Design review of the part built by this model. Coordinates are the model's own, in mm. A direction names the side the tool comes from. Coordinates: 2 decimals unless noted, no trailing zeros. Order: outer loops, then holes, each group sorted by start corner. A loop starts at its lowest first (then second) coordinate and runs counter-clockwise, first axis right, second up. Notation, with made-up numbers: (-38.5, 46.25) - (4.5, 46.25) arc R21 cw to (4.5, 76.25) - close; hole circle Ø6 at (55.5, -20.5). An arc over 180 degrees is marked (long way). Write each question's results on one line, items separated by ' | '. Start each with the question number.
Autodesk Inventor part; units mm, degrees
ref_plane "Work Plane1" through (0, 0, 5) normal (0, 0, 1) x (1, 0, 0)
ref_plane "YZ Plane" through (0, 0, 0) normal (1, 0, 0) x (0, 1, 0)
ref_plane "XZ Plane" through (0, 0, 0) normal (0, 1, 0) x (-1, 0, 0)
sketch "Sketch1" plane through (0, 0, 0) normal (0, 0, 1) x (1, 0, 0)
  line L0 (-5.8474, 0) -> (5.8474, 0) construction
  line L1 (2.5, 18.75) -> (7.5, 18.75)
  line L2 (7.5, 18.75) -> (7.5, 37.5)
  line L3 (7.5, 37.5) -> (-7.5, 37.5)
  line L4 (-7.5, 37.5) -> (-7.5, 18.75)
  line L5 (-7.5, 18.75) -> (2.5, 18.75)
  circle A0 centre (3.75, 33.75) radius 1.6
  circle A1 centre (-3.75, 33.75) radius 1.6
  line L6 (2.5, -18.75) -> (7.5, -18.75)
  line L7 (7.5, -18.75) -> (7.5, -37.5)
  line L8 (7.5, -37.5) -> (-7.5, -37.5)
  line L9 (-7.5, -37.5) -> (-7.5, -18.75)
  line L10 (-7.5, -18.75) -> (2.5, -18.75)
  circle A2 centre (3.75, -33.75) radius 1.6
  circle A3 centre (-3.75, -33.75) radius 1.6
  line L11 (7.5, 28.125) -> (27.5, 8.125)
  line L12 (7.5, 28.125) -> (35.7843, 28.125) construction
  line L13 (2.5, 18.75) -> (12.5, 8.75)
  line L14 (12.5, 8.75) -> (12.5, 0)
  line L15 (27.5, 8.125) -> (27.5, 0)
  line L16 (7.5, -28.125) -> (27.5, -8.125)
  line L17 (2.5, -18.75) -> (12.5, -8.75)
  line L18 (12.5, -8.75) -> (12.5, 0)
  line L19 (27.5, -8.125) -> (27.5, 0)
  point P0 (0, 0)
  point P1 (0, 0)
  point P2 (2.5, -18.75)
  point P3 (2.5, -18.75)
  point P4 (2.5, 18.75)
  dimension "d2" = 15
  dimension "d3" = 18.75
  dimension "d4" = 7.5
  dimension "d5" = 3.2
  dimension "d6" = 3.2
  dimension "d7" = 3.75
  dimension "d8" = 3.75
  dimension "d9" = 7.5
  dimension "d10" = 18.75
  dimension "d20" = 45
  dimension "d21" = 20
  dimension "d31" = 20
  dimension "d32" = 10
ref_plane "Work Plane1" through (0, 0, 5) normal (0, 0, 1) x (1, 0, 0)
extrude "Extrusion3" add sketch "Sketch1" along normal blind 5
chamfer "Chamfer4" distance 0.4 angle 45 4 edges at (2.15, 33.75, 5) (-5.35, 33.75, 5) (2.15, -33.75, 5) (-5.35, -33.75, 5)
sketch "Sketch4" plane through (0, 0, 5) normal (0, 0, 1) x (1, 0, 0)
  circle A0 centre (20, 0) radius 5
  line L0 (27.5, -8.125) -> (27.5, 8.125)
  line L1 (12.5, 8.75) -> (12.5, -8.75)
  point P0 (0, 0)
  point P1 (12.5, 0)
  dimension "d40" = 10
  dimension "d41" = 15
  dimension "d42" = 7.5
extrude "Extrusion5" cut sketch "Sketch4" against normal blind 5
chamfer "Chamfer5" distance 0.4 angle 45 1 edges at (15, 0, 5)
sketch "Sketch5" plane through (0, 0, 0) normal (0, 0, -1) x (-1, 0, 0)
  circle A0 centre (-20, 0) radius 5
  circle A1 centre (-20, 0) radius 5
  circle A2 centre (-20, 0) radius 6
  point P0 (0, 0)
  dimension "d48" = 12
extrude "Extrusion6" add sketch "Sketch5" along normal blind 6.5
chamfer "Chamfer6" distance 1 angle 45 2 edges at (7.5, 37.5, 2.5) (7.5, -37.5, 2.5)
equation "\"d7\" = 0.25 * d2"
equation "\"d8\" = d7"
equation "\"d9\" = 0.5 * d2"
equation "\"d31\" = d21"
properties part number "uchwyt-GM" material "Stainless Steel"
(1) Take a section at D-D (z = -2). State the section outline as (x, y) points, plus the area to 3 significant figures.
(2) Take a section at C-C (y = 33.75). State the section outline as (x, z) points, plus the area to 3 significant figures.
(3) Tool access review of faces 4 (the face through (7.5, -32, 2)), 5 (the face through (7.43, -13.82, 2.46)), 6 (the face through (7.5, 32, 2)): name each direction out of +Z, -Z, +X, -X, +Y, -Y from which nothing blocks a thin tool from reaching the whole face with its end or side.
(4) Clearance check with flat-ended pins moving along their axes: pin 1 (6 mm diameter, centred on x = 12, y = 5.5, fed in from -Z); pin 2 (1.5 mm diameter, centred on y = 31, z = 2.5, fed in from +X); pin 3 (2 mm diameter, centred on y = -10, z = -1.5, fed in from +X); pin 4 (3 mm diameter, centred on x = 19.5, z = -4.5, fed in from +Y). State where each tip first meets the part, or that it passes through.
(5) Take a section at A-A (x = -3.75). State the section outline as (y, z) points, plus the area to 3 significant figures.
(6) Take a section at B-B (y = 0). State the section outline as (x, z) points, plus the area to 3 significant figures.
(7) Mouldability with a two-part tool opening along X and no side actions: class faces 1 (the face through (27.5, 0, 2)), 2 (the face through (-3, -18.75, 2)), 3 (the face through (4.49, 35.17, 2.27)) as +X half, -X half, draft (parallel to the pull), parting line (faces both ways), or undercut.
(8) To check wall thickness, follow line 1 along Y through (x, z) = (-3.75, 3.3); line 2 along Y through (x, z) = (4.5, 3.25); line 3 along Y through (x, z) = (-1, 0.5). State the ranges of each line that lie inside material, in increasing order. Write a range as [from, to].
Worked out:
1) outline: circle Ø12 at (20, 0); hole circle Ø10 at (20, 0) | area: 34.6 mm^2
2) outline: (-7.5, 0) - (-5.35, 0) - (-5.35, 4.6) - (-5.75, 5) - (-7.5, 5) - close; (-2.15, 0) - (2.15, 0) - (2.15, 4.6) - (1.75, 5) - (-1.75, 5) - (-2.15, 4.6) - close; (5.35, 0) - (7.5, 0) - (7.5, 5) - (5.75, 5) - (5.35, 4.6) - close | area: 42.7 mm^2
3) face 4: +Z, -Z, +X, -Y | face 5: +Z, -Z, -X | face 6: +Z, -Z, +X, +Y
4) pin 1: z = 0 | pin 2: x = 7.5 | pin 3: through | pin 4: y = 6
5) outline: (-37.5, 0) - (-35.35, 0) - (-35.35, 4.6) - (-35.75, 5) - (-37.5, 5) - close; (-32.15, 0) - (-18.75, 0) - (-18.75, 5) - (-31.75, 5) - (-32.15, 4.6) - close; (18.75, 0) - (32.15, 0) - (32.15, 4.6) - (31.75, 5) - (18.75, 5) - close; (35.35, 0) - (37.5, 0) - (37.5, 5) - (35.75, 5) - (35.35, 4.6) - close | area: 155 mm^2
6) outline: (12.5, 0) - (14, 0) - (14, -6.5) - (15, -6.5) - (15, 4.6) - (14.6, 5) - (12.5, 5) - close; (25, -6.5) - (26, -6.5) - (26, 0) - (27.5, 0) - (27.5, 5) - (25.4, 5) - (25, 4.6) - close | area: 37.8 mm^2
7) face 1: +X half | face 2: draft | face 3: undercut
8) line 1: [-37.5, -35.35], [-32.15, -18.75], [18.75, 32.15], [35.35, 37.5] | line 2: [-37.5, -35.16], [-32.34, -16.75], [16.75, 32.34], [35.16, 37.5] | line 3: [-37.5, -18.75], [18.75, 37.5]
